```python
from build123d import *

# Parameters (mm, degrees)
EXTRUDE_1_DEPTH     = 150
SKETCH_2_R          = 3
CUT_EXTRUDE_1_DEPTH = 300
SKETCH_3_W          = 40
SKETCH_3_H          = 33
CUT_EXTRUDE_2_DEPTH = 10
FILLET_1_R          = 15


with BuildPart() as part:
    # 草图1 → 凸台-拉伸1 (new body)
    with BuildSketch(Plane(origin=(0, 0, 0), x_dir=(0, 0, -1), z_dir=(1, 0, 0))):
        Polygon((-16.5, 4), (-16.5, 34), (-20.5, 34), (-20.5, 0), (0, 0), (0, 4), align=None)
        Polygon((16.5, 4), (0, 4), (0, 0), (20.5, 0), (20.5, 34), (16.5, 34), align=None)
    extrude(amount=EXTRUDE_1_DEPTH)

    # 草图2 → 切除-拉伸1 (cut)
    with BuildSketch(Plane.XY.offset(20.5)):
        with Locations(Location((15, 19, 0), (0, 0, 90))):
            Circle(SKETCH_2_R)
        with Locations(Location((135, 19, 0), (0, 0, 90))):
            Circle(SKETCH_2_R)
    extrude(amount=-CUT_EXTRUDE_1_DEPTH, mode=Mode.SUBTRACT)

    # 草图3 → 切除-拉伸2 (cut)
    with BuildSketch(Plane.XZ):
        with Locations((130, 0)):
            Rectangle(SKETCH_3_W, SKETCH_3_H)
        with Locations((20, 0)):
            Rectangle(SKETCH_3_W, SKETCH_3_H)
    extrude(amount=-CUT_EXTRUDE_2_DEPTH, mode=Mode.SUBTRACT)

    # 圆角1
    fillet_1_edges = [part.edges().sort_by_distance(p)[0] for p in [
        (0, 0, 18.5),
        (0, 34, 18.5),
        (150, 34, 18.5),
        (150, 0, 18.5),
        (150, 34, -18.5),
        (150, 0, -18.5),
        (0, 0, -18.5),
        (0, 34, -18.5),
    ]]
    fillet(fillet_1_edges, radius=FILLET_1_R)


solid = part.part
```
Model file for the job. Use its own axes, mm. A direction names the side the tool comes from. Coordinates: 2 decimals unless noted, no trailing zeros. Loops run counter-clockwise (first coordinate to the right, second up) from the corner with the lowest first, then second, coordinate; pieces in that order, holes last. Notation, with made-up numbers: (-28, -36.75) - (22, -36.75) arc R30 cw to (22, -5.75) - close; hole circle Ø9 at (6, 29). An arc over 180 degrees is marked (long way). Write item = value, one per line. Start each with the question number.
Item 1: Saw through at C-C, the plane z = 14. List the corners of the cut face in (x, y), then the cut area to 3 significant figures.
Item 2: Drop flat-ended pins along their axis: pin 1 Ø3.5 at (x, y) = (135, 19) entering from -Z; pin 2 Ø3 at (y, z) = (1.5, 1.5) entering from +X; pin 3 Ø4 at (x, z) = (100.5, 0) entering from +Y; pin 4 Ø12 at (y, z) = (6.5, -5) entering from -X. Give the stop position or say it passes through.
Item 3: Pull direction Y, two halves, no side cores. Call faces 1 (the face through (0, 17, 19)), 2 (the face through (4.51, 4.28, 18.47)), 3 (the face through (17.93, 18.35, 18.53)): +Y half, -Y half, draft (parallel to the pull), parting line (faces both ways), or undercut.
Item 4: Wall check: probe 1 along Y at (x, z) = (135, 18.05); probe 2 along Z at (x, y) = (120.5, 27); probe 3 along Y at (x, z) = (47, 6). Give the ranges that are in metal, low to high. Write a range as [from, to].
Item 5: Saw through at B-B, the plane x = 102.5. List the corners of the cut face in (y, z), then the cut area to 3 significant figures.
Item 6: Saw through at A-A, the plane y = 6. List the corners of the cut face in (x, z).
Item 7: Saw through at D-D, the plane y = 32.5. List the corners of the cut face in (x, z).
Item 8: 3-axis set-ups, long thin cutter, end or side, ignore diameter. For faces 4 (the face through (110, 2, 0)), 5 (the face through (75, 4, 0)), 6 (the face through (74, 0, 0)): which of +Z, -Z, +X, -X, +Y, -Y reach the whole face in a straight line?
Answers:
q1.outline = (40, 0) - (110, 0) - (110, 4) - (40, 4) - close
q1.area = 280 mm2
q2.pin_1 = through
q2.pin_2 = 110
q2.pin_3 = 4
q2.pin_4 = 40
q3.face_1 = draft
q3.face_2 = -Y half
q3.face_3 = undercut
q4.probe_1 = [0, 16], [22, 34]
q4.probe_2 = [-20.5, -16.5], [16.5, 20.5]
q4.probe_3 = [0, 4]
q5.outline = (0, -20.5) - (34, -20.5) - (34, -16.5) - (4, -16.5) - (4, 16.5) - (34, 16.5) - (34, 20.5) - (0, 20.5) - close
q5.area = 404 mm2
q6.outline = (3, -20.5) - (147, -20.5) - (147, -16.5) - (3, -16.5) - close; (3, 16.5) - (147, 16.5) - (147, 20.5) - (3, 20.5) - close
q7.outline = (8.46, -20.5) - (141.54, -20.5) - (141.54, -16.5) - (8.46, -16.5) - close; (8.46, 16.5) - (141.54, 16.5) - (141.54, 20.5) - (8.46, 20.5) - close
q8.face_4 = +X, +Y, -Y
q8.face_5 = +X, -X, +Y
q8.face_6 = +Z, -Z, +X, -X, -Y
